from build123d import *

# Parameters (mm, degrees)
F0_W     = 88
F0_H     = 10
F1_DEPTH = 23
F2_R     = 3.6
F3_DEPTH = 22
F4_R     = 4.99999


# Not quite as in the source:
# - a fillet or chamfer is up to 0.001 mm smaller than in the source, because OpenCascade refuses the exact size


with BuildPart() as f1:
    # F0 (on Top) → F1 (new body)
    with BuildSketch(Plane.XY):
        Rectangle(F0_W, F0_H)
    extrude(amount=F1_DEPTH)

    # F2 (on face) → F3 (cut)
    with BuildSketch(Plane.XY.offset(23)):
        with Locations((-38.25, 0)):
            Circle(F2_R)
        with Locations((-29.75, 0)):
            Circle(F2_R)
        with Locations((-21.25, 0)):
            Circle(F2_R)
        with Locations((-12.75, 0)):
            Circle(F2_R)
        with Locations((-4.25, 0)):
            Circle(F2_R)
        with Locations((4.25, 0)):
            Circle(F2_R)
        with Locations((12.75, 0)):
            Circle(F2_R)
        with Locations((21.25, 0)):
            Circle(F2_R)
        with Locations((29.75, 0)):
            Circle(F2_R)
        with Locations((38.25, 0)):
            Circle(F2_R)
    extrude(amount=-F3_DEPTH, mode=Mode.SUBTRACT)

    # F4 (radius 5 in the source; OpenCascade refuses exactly that, so slightly less here)
    f4_edges = [f1.edges().sort_by_distance(p)[0] for p in [
        (44, 5, 11.5),
        (44, -5, 11.5),
        (-44, -5, 11.5),
        (-44, 5, 11.5),
    ]]
    fillet(f4_edges, radius=F4_R)


solid = f1.part
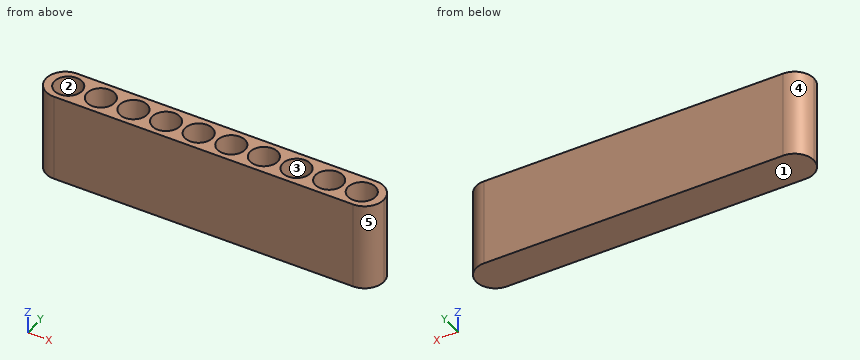
For this review, take the finished solid that the model builds, in its own axes (mm). Face numbers are marked on the shaded views. A direction names the side the tool comes from. Coordinates: 2 decimals unless noted, no trailing zeros. Order: outer loops, then holes, each group sorted by start corner. A loop starts at its lowest first (then second) coordinate and runs counter-clockwise, first axis right, second up. Notation, with made-up numbers: (-8, -16) - (-3, -16) arc R26 ccw to (-3, -1) - close; hole circle Ø9 at (40.5, -26). An arc over 180 degrees is marked (long way). Use one line per item in the form item = value.
Q1. For probe 1 along Y at (x, z) = (29.75, 14); probe 2 along Z at (x, y) = (6, 0.25); probe 3 along Y at (x, z) = (27.5, 7.5), list the stretches that pass through material, from the lowest coordinate up. Write a range as from..to.
Checked values:
probe_1 = -5..-3.6, 3.6..5
probe_2 = 0..1
probe_3 = -5..-2.81, 2.81..5
Q2. For the marked faces 1 and 2, list the 3-axis set-ups (+Z, -Z, +X, -X, +Y, -Y) from which the entire face can be reached by the end or side of a thin tool; tool diameter is ignored.
Checked values:
face_1 = -Z, +X, -X, +Y, -Y
face_2 = +Z
Q3. Consider section C-C (x = 28). Give the boundary of the cut face in (y, z), then the cut area to 3 significant figures.
Checked values:
outline = (-5, 0) - (5, 0) - (5, 23) - (3.15, 23) - (3.15, 1) - (-3.15, 1) - (-3.15, 23) - (-5, 23) - close
area = 91.6 mm2
Q4. Consider section A-A (z = 4). Give the number of separate pieces and of enclosed holes in the cut face, then the cut area to 3 significant figures.
Checked values:
separate_pieces = 1
enclosed_holes = 10
area = 451 mm2
Q5. Consider section B-B (x = -21.25). Give the boundary of the cut face in (y, z), then the cut area to 3 significant figures.
Checked values:
outline = (-5, 0) - (5, 0) - (5, 23) - (3.6, 23) - (3.6, 1) - (-3.6, 1) - (-3.6, 23) - (-5, 23) - close
area = 71.6 mm2
Q6. Draft analysis for pull direction X (two halves, no side actions). For the marked faces 3, 4 and 5, state which applies: +X half, -X half, draft (parallel to the pull), parting line (faces both ways), or undercut.
Checked values:
face_3 = undercut
face_4 = -X half
face_5 = +X half
Q7. For P1, Ø6, axis at x = 23, y = 0, coming from the +Z side; P2, Ø6, axis at x = 38.25, y = 0, coming from the +Z side, all flat-tipped, find the tip position at first contact; note any pin that passes through.
Checked values:
P1 = 23
P2 = 1
